from build123d import *

# Parameters (mm, degrees)
SKETCH_1_R           = 5
EXTRUDE_1_DEPTH      = 10.5
EXTRUDE_1_DEPTH_BACK = 10.5
EXTRUDE_3_DEPTH      = 4.5
EXTRUDE_3_DEPTH_BACK = 4.5
SKETCH_7_R           = 6
EXTRUDE_4_DEPTH      = 3
SKETCH_8_R           = 6
EXTRUDE_5_DEPTH      = 3
SKETCH_9_R           = 9.5
CUT_EXTRUDE_1_DEPTH  = 7
SKETCH_10_R          = 8.5
CUT_EXTRUDE_2_DEPTH  = 9
SKETCH_13_W          = 25
SKETCH_13_H          = 45
CUT_EXTRUDE_3_DEPTH  = 2


with BuildPart() as part:
    # Sketch 1 → Extrude 1 (new body, two sides)
    with BuildSketch(Plane(origin=(0, 0, 0), x_dir=(1, 0, 0), z_dir=(0, 1, 0))) as extrude_1_sk:
        Circle(SKETCH_1_R)
    extrude(amount=EXTRUDE_1_DEPTH)
    extrude(extrude_1_sk.sketch, amount=-EXTRUDE_1_DEPTH_BACK)

    # Sketch 6 → Extrude 3 (add, two sides)
    with BuildSketch(Plane(origin=(0, 0, 0), x_dir=(1, 0, 0), z_dir=(0, 1, 0))) as extrude_3_sk:
        with BuildLine():
            Line((-12.5, 0), (-12.5, -260))
            ThreePointArc((-12.5, -260), (0, -272.5), (12.5, -260))
            Line((12.5, -260), (12.5, 0))
            ThreePointArc((12.5, 0), (0, 12.5), (-12.5, 0))
        make_face()
    extrude(amount=EXTRUDE_3_DEPTH)
    extrude(extrude_3_sk.sketch, amount=-EXTRUDE_3_DEPTH_BACK)

    # Sketch 7 → Extrude 4 (add)
    with BuildSketch(Plane.XZ.offset(4.5)):
        Circle(SKETCH_7_R)
    extrude(amount=EXTRUDE_4_DEPTH)

    # Sketch 8 → Extrude 5 (add)
    with BuildSketch(Plane(origin=(0, 4.5, 0), x_dir=(1, 0, 0), z_dir=(0, 1, 0))):
        Circle(SKETCH_8_R)
    extrude(amount=EXTRUDE_5_DEPTH)

    # Sketch 9 → Cut-Extrude 1 (cut)
    with BuildSketch(Plane.XZ.offset(4.5)):
        with Locations((0, 250)):
            Circle(SKETCH_9_R)
    extrude(amount=-CUT_EXTRUDE_1_DEPTH, mode=Mode.SUBTRACT)

    # Sketch 10 → Cut-Extrude 2 (cut, through all)
    with BuildSketch(Plane.XZ.offset(-2.5)):
        with Locations((0, 250)):
            Circle(SKETCH_10_R)
    extrude(amount=-CUT_EXTRUDE_2_DEPTH, mode=Mode.SUBTRACT)

    # Sketch 13 → Cut-Extrude 3 (cut)
    with BuildSketch(Plane.XZ.offset(4.5)):
        with Locations((0, 250)):
            Rectangle(SKETCH_13_W, SKETCH_13_H)
    extrude(amount=-CUT_EXTRUDE_3_DEPTH, mode=Mode.SUBTRACT)


solid = part.part
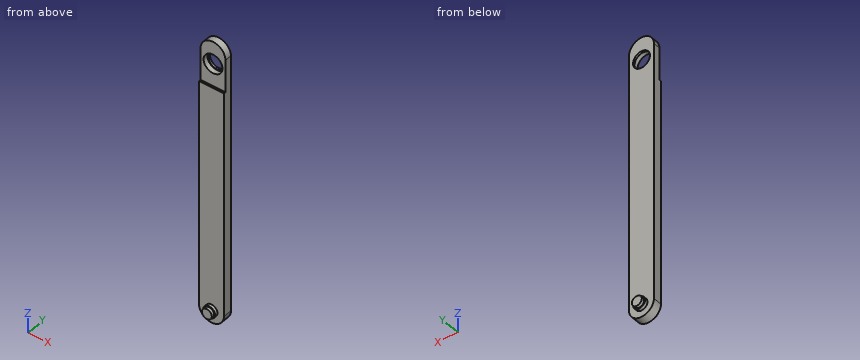
Input: part model. Units: mm. Frame: model coordinates. Give positions to 0.01 mm unless a question says otherwise; leave off trailing zeros. Order: outer loops, then holes, each group sorted by start corner. A loop starts at its lowest first (then second) coordinate and runs counter-clockwise, first axis right, second up. Notation, with made-up numbers: (-5.75, 27) - (12.25, 27) arc R28 cw to (12.25, 61) - close; hole circle Ø4 at (21, 71). An arc over 180 degrees is marked (long way). Write each question's results on one line, items separated by ' | '.
Item 1: Material intervals for line 1 along Z through (x, y) = (0, 3.4); line 2 along Z through (x, y) = (0, -0.5); line 3 along Y through (x, z) = (8.75, 22), sorted ascending.
A:
line 1: z = -12.5 to 241.5, 258.5 to 272.5 | line 2: z = -12.5 to 240.5, 259.5 to 272.5 | line 3: y = -4.5 to 4.5
Item 2: Section A-A (z = 250). Return loops of the section in (x, y).
A:
outline: (-12.5, -2.5) - (-9.5, -2.5) - (-9.5, 2.5) - (-8.5, 2.5) - (-8.5, 4.5) - (-12.5, 4.5) - close; (8.5, 2.5) - (9.5, 2.5) - (9.5, -2.5) - (12.5, -2.5) - (12.5, 4.5) - (8.5, 4.5) - close
Item 3: Contact query for flat-ended pins moving along their axis: pin 1 Ø12 at (x, z) = (-5, 207.5) entering from +Y; pin 2 Ø2 at (x, y) = (4.5, 6.5) entering from +Z; pin 3 Ø7.5 at (x, z) = (0.5, 260.5) entering from -Y. Output: stop coordinate, or through.
A:
pin 1: stops at y = 4.5 | pin 2: stops at z = 4.87 | pin 3: stops at y = -2.5
Item 4: Section C-C (z = 97.5). Return loops of the section in (x, y), and give its area (3 significant figures).
A:
outline: (-12.5, -4.5) - (12.5, -4.5) - (12.5, 4.5) - (-12.5, 4.5) - close | area: 225 mm^2
